```python
from build123d import *

# Parameters (mm, degrees)
SKETCH1_R           = 152.5
SKETCH1_R_2         = 2
SKETCH1_R_3         = 10
SKETCH1_R_4         = 8
SKETCH1_R_5         = 4.5
BOSS_EXTRUDE1_DEPTH = 2.15


with BuildPart() as part:
    # Sketch1 → Boss-Extrude1 (new body)
    with BuildSketch(Plane(origin=(0, 0, 0), x_dir=(1, 0, 0), z_dir=(0, 1, 0))):
        Circle(SKETCH1_R)
        with Locations((-25, -136.224997706)):
            Circle(SKETCH1_R_2, mode=Mode.SUBTRACT)
        with Locations((-25, -122.724997706)):
            Circle(SKETCH1_R_2, mode=Mode.SUBTRACT)
        with Locations((25, -136.224997706)):
            Circle(SKETCH1_R_2, mode=Mode.SUBTRACT)
        with Locations((25, -122.724997706)):
            Circle(SKETCH1_R_2, mode=Mode.SUBTRACT)
        with Locations((-118.782965693, -39.711863758)):
            Circle(SKETCH1_R_2, mode=Mode.SUBTRACT)
        with Locations((-130.474308644, -46.461863758)):
            Circle(SKETCH1_R_2, mode=Mode.SUBTRACT)
        with Locations((-93.782965693, -83.013133948)):
            Circle(SKETCH1_R_2, mode=Mode.SUBTRACT)
        with Locations((-105.474308644, -89.763133948)):
            Circle(SKETCH1_R_2, mode=Mode.SUBTRACT)
        with Locations((-93.782965693, 83.013133948)):
            Circle(SKETCH1_R_2, mode=Mode.SUBTRACT)
        with Locations((-105.474308644, 89.763133948)):
            Circle(SKETCH1_R_2, mode=Mode.SUBTRACT)
        with Locations((-118.782965693, 39.711863758)):
            Circle(SKETCH1_R_2, mode=Mode.SUBTRACT)
        with Locations((-130.474308644, 46.461863758)):
            Circle(SKETCH1_R_2, mode=Mode.SUBTRACT)
        with Locations((25, 122.724997706)):
            Circle(SKETCH1_R_2, mode=Mode.SUBTRACT)
        with Locations((25, 136.224997706)):
            Circle(SKETCH1_R_2, mode=Mode.SUBTRACT)
        with Locations((-25, 122.724997706)):
            Circle(SKETCH1_R_2, mode=Mode.SUBTRACT)
        with Locations((-25, 136.224997706)):
            Circle(SKETCH1_R_2, mode=Mode.SUBTRACT)
        with Locations((118.782965693, 39.711863758)):
            Circle(SKETCH1_R_2, mode=Mode.SUBTRACT)
        with Locations((130.474308644, 46.461863758)):
            Circle(SKETCH1_R_2, mode=Mode.SUBTRACT)
        with Locations((93.782965693, 83.013133948)):
            Circle(SKETCH1_R_2, mode=Mode.SUBTRACT)
        with Locations((105.474308644, 89.763133948)):
            Circle(SKETCH1_R_2, mode=Mode.SUBTRACT)
        with Locations((93.782965693, -83.013133948)):
            Circle(SKETCH1_R_2, mode=Mode.SUBTRACT)
        with Locations((105.474308644, -89.763133948)):
            Circle(SKETCH1_R_2, mode=Mode.SUBTRACT)
        with Locations((118.782965693, -39.711863758)):
            Circle(SKETCH1_R_2, mode=Mode.SUBTRACT)
        with Locations((130.474308644, -46.461863758)):
            Circle(SKETCH1_R_2, mode=Mode.SUBTRACT)
        with Locations((0, -100.224997706)):
            Circle(SKETCH1_R_3, mode=Mode.SUBTRACT)
        with Locations((-86.797394108, 50.112498853)):
            Circle(SKETCH1_R_3, mode=Mode.SUBTRACT)
        with Locations((86.797394108, 50.112498853)):
            Circle(SKETCH1_R_3, mode=Mode.SUBTRACT)
        with Locations((54.5, -122.724997706)):
            Circle(SKETCH1_R_4, mode=Mode.SUBTRACT)
        with Locations((-50, 61.116126736)):
            Circle(SKETCH1_R_5, mode=Mode.SUBTRACT)
        with Locations((-50, -38.883873264)):
            Circle(SKETCH1_R_5, mode=Mode.SUBTRACT)
        with Locations((50, -38.883873264)):
            Circle(SKETCH1_R_5, mode=Mode.SUBTRACT)
        with Locations((50, 61.116126736)):
            Circle(SKETCH1_R_5, mode=Mode.SUBTRACT)
        with BuildLine():
            Line((-23.75, 61.525), (23.75, 61.525))
            ThreePointArc((23.75, 61.525), (32.775, 52.5), (23.75, 43.475))
            Line((23.75, 43.475), (-23.75, 43.475))
            ThreePointArc((-23.75, 43.475), (-32.775, 52.5), (-23.75, 61.525))
        make_face(mode=Mode.SUBTRACT)
        with BuildLine():
            Line((-62, -125.799997706), (-62, -119.649997706))
            ThreePointArc((-62, -119.649997706), (-54.5, -115.126660151), (-47, -119.649997706))
            Line((-47, -119.649997706), (-47, -125.799997706))
            ThreePointArc((-47, -125.799997706), (-54.5, -130.323335261), (-62, -125.799997706))
        make_face(mode=Mode.SUBTRACT)
    extrude(amount=BOSS_EXTRUDE1_DEPTH)


solid = part.part
```
Read the model definition and answer for the solid it produces. Units are mm, in the model's axes. A direction names the side the tool comes from. Give positions to 0.01 mm unless a question says otherwise; leave off trailing zeros. Order: outer loops, then holes, each group sorted by start corner. A loop starts at its lowest first (then second) coordinate and runs counter-clockwise, first axis right, second up. Notation, with made-up numbers: (78.25, 8) -> (114.25, 8) arc R19 ccw to (114.25, 43) -> close; hole circle Ø6 at (-13.75, -30). An arc over 180 degrees is marked (long way). Write item = value, one per line.
1. For faces 1 (the face through (-2, 2.15, -2)), 2 (the face through (32.773, 1.06, -52.698)), determine the directions among +Z, -Z, +X, -X, +Y, -Y from which every point of the face is accessible in a straight line to the end or side of a thin tool.
Numbers:
face_1 = +Z, -Z, +X, -X, +Y
face_2 = +Y, -Y
2. A cutting plane is placed at D-D, the plane z = -27. Write down the section's boundary in (x, y).
Numbers:
outline = (-150.09, 0) -> (150.09, 0) -> (150.09, 2.15) -> (-150.09, 2.15) -> close
3. Given pin 1 (18 mm diameter, centred on x = -86.8, z = -50.11, fed in from -Y), flat-ended and moving along its own axis, determine where the tip first touches the part or whether it passes through.
Numbers:
pin_1 = through
4. Straight lines are drawn through the part: line 1 along Z through (x, y) = (92, 1.05); line 2 along Z through (x, y) = (106.5, 1.6); line 3 along Z through (x, y) = (25, 0.6) (3 decimals). For each, find the intervals that lie inside material, in ascending order.
Numbers:
line_1 = -121.62 to -83.92, -82.11 to -58.65, -41.57 to 82.11, 83.92 to 121.62
line_2 = -109.15 to -91.48, -88.05 to 88.05, 91.48 to 109.15
line_3 = -150.437 to -138.225, -134.225 to -124.725, -120.725 to -61.438, -43.562 to 120.725, 124.725 to 134.225, 138.225 to 150.437
5. The mould has two halves that part along X. Classify faces 3 (the face through (-152.353, 1.06, -6.705)), 4 (the face through (-45.71, 1.06, -62.47)), 5 (the face through (-2, 0, -2)), 6 (the face through (-1.3, 1.06, 90.31)): +X half, -X half, draft (parallel to the pull), parting line (faces both ways), or undercut.
Numbers:
face_3 = parting line
face_4 = undercut
face_5 = draft
face_6 = undercut
6. A cutting plane is placed at B-B, the plane x = 50. Write down the section's boundary in (y, z), and give its area (3 significant figures).
Numbers:
outline = (0, -144.07) -> (2.15, -144.07) -> (2.15, -65.62) -> (0, -65.62) -> close; (0, -56.62) -> (2.15, -56.62) -> (2.15, 34.38) -> (0, 34.38) -> close; (0, 43.38) -> (2.15, 43.38) -> (2.15, 116.11) -> (0, 116.11) -> close; (0, 129.34) -> (2.15, 129.34) -> (2.15, 144.07) -> (0, 144.07) -> close
area = 552 mm²
7. A cutting plane is placed at C-C, the plane y = 1.4. Count the separate pieces of the cut face and the enclosed holes in it, and give its area (3 significant figures).
Numbers:
separate_pieces = 1
enclosed_holes = 34
area = 70,100 mm²
8. A cutting plane is placed at A-A, the plane x = 0. Write down the section's boundary in (y, z) (3 decimals), and give its area (3 significant figures).
Numbers:
outline = (0, -152.5) -> (2.15, -152.5) -> (2.15, -61.525) -> (0, -61.525) -> close; (0, -43.475) -> (2.15, -43.475) -> (2.15, 90.225) -> (0, 90.225) -> close; (0, 110.225) -> (2.15, 110.225) -> (2.15, 152.5) -> (0, 152.5) -> close
area = 574 mm²
